The model under review builds one solid part; all positions refer to its coordinate system, in mm. A direction names the side the tool comes from. Round coordinates to 2 decimals unless told otherwise and drop trailing zeros. Write each loop counter-clockwise with the first axis right and the second up, starting at its lowest first coordinate (ties: lowest second). Pieces come first, ordered by that corner, then holes. Notation, with made-up numbers: M 12,1.5 L 19,1.5 A21 ccw 19,16.5 Z; hole C 84.25,25.5 d4. An arc over 180 degrees is marked long. Write item = value, one per line. Start each with the question number.
Item 1: Take a section at A-A, the plane z = -8.5. Give the boundary of the cut face in (x, y), plus the area to 3 significant figures.
Item 2: To check wall thickness, follow line 1 along Y through (x, z) = (-3.5, 26.25); line 2 along Z through (x, y) = (-6, 0.25); line 3 along Z through (x, y) = (-3.5, 8). State the ranges of each line that lie inside material, in increasing order.
Item 3: For pin 1 Ø7.5 at (x, y) = (-10.5, 12) entering from -Z; pin 2 Ø0.8 at (y, z) = (11, -5) entering from +X; pin 3 Ø4.5 at (x, y) = (-3.5, 11.5) entering from +Z; pin 4 Ø3 at (x, z) = (-5.5, -14.5) entering from +Y, all flat-tipped, find the tip position at first contact; note any pin that passes through.
Item 4: Tool access review of faces 4 (the flat face through (-9, 11, -18.5)), 5 (the flat face through (-9, 11, 0)), 6 (the flat face through (-6, 2, 0)): name each direction out of +Z, -Z, +X, -X, +Y, -Y from which nothing blocks a thin tool from reaching the whole face with its end or side.
Item 5: The part is to be moulded in two halves that separate along X. For faces 1 (the flat face through (-12, 4, 0)), 2 (the flat face through (-7, 10, -18.5)), 3 (the flat face through (-6, 8, -30)), say which applies: +X half, -X half, draft (parallel to the pull), parting line (faces both ways), or undercut.
from build123d import *

# Parameters (mm, degrees)
EXTRUDE_1_DEPTH          = 30
CUT_EXTRUDE_1_REACH      = 37.944
SKETCH_2_W               = 10
SKETCH_2_H               = 26
HOLE_WIZARD_1_AT_2_COUNT = 2
HOLE_WIZARD_1_AT_2_PITCH = 17
CUT_EXTRUDE_2_DEPTH      = 5


with BuildPart() as part:
    # 草图1 → 凸台-拉伸1 (new, symmetric)
    with BuildSketch(Plane.XY):
        with BuildLine():
            Line((0, 0), (-13, 0))
            ThreePointArc((-13, 0), (-13.707106781, 0.292893219), (-14, 1))
            Line((-14, 1), (-14, 7.559208386))
            ThreePointArc((-14, 7.559208386), (-13.915047807, 7.962553786), (-13.674624977, 8.297369033))
            Line((-13.674624977, 8.297369033), (-6.535812398, 14.821722909))
            ThreePointArc((-6.535812398, 14.821722909), (0.830646134, 10.277091966), (-7.82487065, 10.256821067))
            Line((-7.82487065, 10.256821067), (-6.3347696, 11.618664715))
            ThreePointArc((-6.3347696, 11.618664715), (-6.120158424, 11.654472256), (-5.999856115, 11.47317832))
            ThreePointArc((-5.999856115, 11.47317832), (-1.20700412, 10.503922746), (-5.186562443, 13.345401616))
            Line((-5.186562443, 13.345401616), (-11.674624977, 7.415785805))
            ThreePointArc((-11.674624977, 7.415785805), (-11.915047807, 7.080970558), (-12, 6.677625158))
            Line((-12, 6.677625158), (-12, 2))
            Line((-12, 2), (0, 2))
            Line((0, 2), (0, 0))
        make_face()
    extrude(amount=EXTRUDE_1_DEPTH, both=True)

    # 草图2 → 切除-拉伸1 (cut, up to next)
    with BuildSketch(Plane(origin=(0, 2, 0), x_dir=(1, 0, 0), z_dir=(0, 1, 0)), mode=Mode.PRIVATE) as cut_extrude_1_sk1:
        with Locations((-4, 0)):
            Rectangle(SKETCH_2_W, SKETCH_2_H)
    cut_extrude_1_tool1 = extrude(cut_extrude_1_sk1.sketch, amount=CUT_EXTRUDE_1_REACH, mode=Mode.PRIVATE) & part.part
    add(cut_extrude_1_tool1.solids().sort_by_distance((-4, 2, 0))[0], mode=Mode.SUBTRACT)

    # 草图3 → 打孔尺寸(%根据十字)槽沉头木螺钉的类型1 (revolve, cut)
    with BuildSketch(Plane(origin=(-6, 2, -8.5), x_dir=(0, 0, 1), z_dir=(1, 0, 0))):
        Polygon((0, 0), (0, 2), (2.5, 2), (2.5, 1.25), (3.75, 0), align=None)
    hole_wizard_1 = revolve(axis=Axis((-6, 8.35, -8.5), (0, -1, 0)), mode=Mode.SUBTRACT)

    # 打孔尺寸(%根据十字)槽沉头木螺钉的类型1 at 2: 打孔尺寸(%根据十字)槽沉头木螺钉的类型1 ×2
    with Locations(*[(0, 0, i * HOLE_WIZARD_1_AT_2_PITCH) for i in range(1, HOLE_WIZARD_1_AT_2_COUNT)]):
        add(hole_wizard_1, mode=Mode.SUBTRACT)

    # 草图5 → 切除-拉伸2 (cut)
    with BuildSketch(Plane(origin=(-10.355516916, 11.330791651, 0), x_dir=(0.7381606464067151, 0.6746249773736669, 0), z_dir=(-0.6746249773736669, 0.7381606464067151, 0))):
        Polygon((-3.325375023, 24.5), (4.674624977, 24.5), (4.674624977, 22.5), (9.674624977, 22.5), (9.674624977, 20.5), (4.674624977, 20.5), (4.674624977, 18.5), (-3.325375023, 18.5), align=None)
        Polygon((9.674624977, -22.5), (9.674624977, -20.5), (4.674624977, -20.5), (4.674624977, -18.5), (-3.325375023, -18.5), (-3.325375023, -24.5), (4.674624977, -24.5), (4.674624977, -22.5), align=None)
    extrude(amount=-CUT_EXTRUDE_2_DEPTH, mode=Mode.SUBTRACT)


solid = part.part
Response values:
q1.outline = M -14,1 A1 ccw -13,0 L -8.5,0 L -8.5,0.75 L -9.75,2 L -12,2 L -12,6.68 A1 cw -11.67,7.42 L -9,9.86 L -9,12.57 L -13.67,8.3 A1 ccw -14,7.56 Z; M -3.5,0 L 0,0 L 0,2 L -2.25,2 L -3.5,0.75 Z
q1.area = 38.2 mm2
q2.line_1 = 0 to 2, 7 to 9, 14 to 16
q2.line_2 = -30 to -11, -6 to 6, 11 to 30
q2.line_3 = -30 to -13, 13 to 30
q3.pin_1 = -30
q3.pin_2 = -9
q3.pin_3 = through
q3.pin_4 = 15.97
q4.face_4 = none
q4.face_5 = +X, +Y
q4.face_6 = +Z, -Z, +X
q5.face_1 = +X half
q5.face_2 = undercut
q5.face_3 = draft
